from build123d import *

# Parameters (mm, degrees)
SKETCH_1_W          = 70
SKETCH_1_H          = 30
EXTRUDE_1_DEPTH     = 2
SKETCH_2_R          = 5
EXTRUDE_2_DEPTH     = 4
SKETCH_3_W          = 100
SKETCH_3_H          = 20
EXTRUDE_3_DEPTH     = 4
EXTRUDE_5_DEPTH     = 100
SKETCH_7_W          = 40
SKETCH_7_H          = 30
EXTRUDE_7_DEPTH     = 6
CUT_EXTRUDE_1_REACH = 97
SKETCH_8_R          = 1.5
CUT_EXTRUDE_2_REACH = 95.814
SKETCH_10_R         = 14


with BuildPart() as part:
    # 草图1 → 凸台-拉伸1 (new body)
    with BuildSketch(Plane(origin=(0, 0, 0), x_dir=(1, 0, 0), z_dir=(0, 1, 0))):
        with Locations((35, 15)):
            Rectangle(SKETCH_1_W, SKETCH_1_H)
    extrude(amount=EXTRUDE_1_DEPTH)

    # 草图2 → 凸台-拉伸2 (add)
    with BuildSketch(Plane(origin=(0, 0, 0), x_dir=(1, 0, 0), z_dir=(0, 1, 0))):
        with Locations(Location((5, 25, 0), (0, 0, 90))):
            Circle(SKETCH_2_R)
        with Locations(Location((5, 5, 0), (0, 0, 270))):
            Circle(SKETCH_2_R)
        with Locations(Location((65, 25, 0), (0, 0, 90))):
            Circle(SKETCH_2_R)
        with Locations(Location((65, 5, 0), (0, 0, 270))):
            Circle(SKETCH_2_R)
    extrude(amount=EXTRUDE_2_DEPTH)

    # 草图3 → 凸台-拉伸3 (add)
    with BuildSketch(Plane(origin=(0, 0, -30), x_dir=(-1, 0, 0), z_dir=(0, 0, -1))):
        with Locations((-35, -10)):
            Rectangle(SKETCH_3_W, SKETCH_3_H)
    extrude(amount=-EXTRUDE_3_DEPTH)

    # 草图5 → 凸台-拉伸5 (add)
    with BuildSketch(Plane.ZY.offset(15)):
        Polygon((-30, 0), (-35, -10), (-30, -20), align=None)
    extrude(amount=-EXTRUDE_5_DEPTH)

    # 草图7 → 凸台-拉伸7 (add)
    with BuildSketch(Plane.XY.offset(-11)):
        with Locations((35, -15)):
            Rectangle(SKETCH_7_W, SKETCH_7_H)
    extrude(amount=EXTRUDE_7_DEPTH)

    # 草图8 → 切除-拉伸1 (cut, up to next)
    with BuildSketch(Plane.XY.offset(-5), mode=Mode.PRIVATE) as cut_extrude_1_sk1:
        with Locations((23, -3)):
            Circle(SKETCH_8_R)
    cut_extrude_1_tool1 = extrude(cut_extrude_1_sk1.sketch, amount=-CUT_EXTRUDE_1_REACH, mode=Mode.PRIVATE) & part.part
    # 草图8 → 切除-拉伸1 (cut, up to next)
    with BuildSketch(Plane.XY.offset(-5), mode=Mode.PRIVATE) as cut_extrude_1_sk2:
        with Locations((47, -3)):
            Circle(SKETCH_8_R)
    cut_extrude_1_tool2 = extrude(cut_extrude_1_sk2.sketch, amount=-CUT_EXTRUDE_1_REACH, mode=Mode.PRIVATE) & part.part
    # 草图8 → 切除-拉伸1 (cut, up to next)
    with BuildSketch(Plane.XY.offset(-5), mode=Mode.PRIVATE) as cut_extrude_1_sk3:
        with Locations((23, -27)):
            Circle(SKETCH_8_R)
    cut_extrude_1_tool3 = extrude(cut_extrude_1_sk3.sketch, amount=-CUT_EXTRUDE_1_REACH, mode=Mode.PRIVATE) & part.part
    # 草图8 → 切除-拉伸1 (cut, up to next)
    with BuildSketch(Plane.XY.offset(-5), mode=Mode.PRIVATE) as cut_extrude_1_sk4:
        with Locations((47, -27)):
            Circle(SKETCH_8_R)
    cut_extrude_1_tool4 = extrude(cut_extrude_1_sk4.sketch, amount=-CUT_EXTRUDE_1_REACH, mode=Mode.PRIVATE) & part.part
    add(cut_extrude_1_tool1.solids().sort_by_distance((23, -3, -5))[0], mode=Mode.SUBTRACT)
    add(cut_extrude_1_tool2.solids().sort_by_distance((47, -3, -5))[0], mode=Mode.SUBTRACT)
    add(cut_extrude_1_tool3.solids().sort_by_distance((23, -27, -5))[0], mode=Mode.SUBTRACT)
    add(cut_extrude_1_tool4.solids().sort_by_distance((47, -27, -5))[0], mode=Mode.SUBTRACT)

    # 草图10 → 切除-拉伸2 (cut, up to next)
    with BuildSketch(Plane.XY.offset(-26), mode=Mode.PRIVATE) as cut_extrude_2_sk1:
        with Locations((35, -15)):
            Circle(SKETCH_10_R)
    cut_extrude_2_tool1 = extrude(cut_extrude_2_sk1.sketch, amount=-CUT_EXTRUDE_2_REACH, mode=Mode.PRIVATE) & part.part
    add(cut_extrude_2_tool1.solids().sort_by_distance((35, -15, -26))[0], mode=Mode.SUBTRACT)


solid = part.part
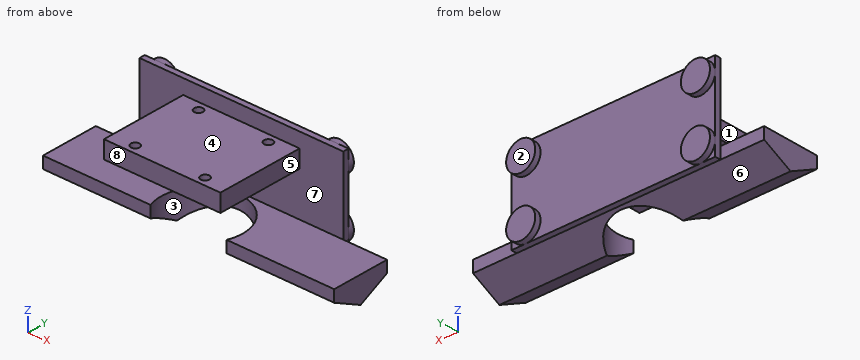
Verification items for the finished model (mm, model axes). Face numbers are marked on the shaded views. A direction names the side the tool comes from. Round coordinates to 2 decimals unless told otherwise and drop trailing zeros. Loops run counter-clockwise (first coordinate to the right, second up) from the corner with the lowest first, then second, coordinate; pieces in that order, holes last. Notation, with made-up numbers: (41.5, -26.5) - (65.5, -26.5) arc R21 cw to (65.5, 5.5) - close; hole circle Ø1 at (70, 1). An arc over 180 degrees is marked (long way). Use one line per item in the form item = value.
1. Section check C-C on x = 27. Record the cut outline in (y, z).
A:
outline = (-30, -11) - (0, -11) - (0, -26) - (-3.51, -26) - (-3.51, -31.76) - (0, -30) - (2, -30) - (2, 0) - (0, 0) - (0, -5) - (-30, -5) - close
2. Gauge pin test, flat ends, axial feed: pin 1 Ø6 at (x, z) = (23, -4) entering from +Y; pin 2 Ø12 at (x, z) = (18, -30) entering from -Y; pin 3 Ø2 at (x, z) = (-11, -28.5) entering from +Y. Record the tip position at first contact, or that the pin passes through.
A:
pin_1 = 2
pin_2 = -20
pin_3 = 0
3. Draft check along Z on the marked faces 6, 7 and 8. Enter one of: pulls with the +Z half, pulls with the -Z half, needs draft (parallel to the pull), parting line crosses it, or undercut.
A:
face_6 = pulls with the -Z half
face_7 = undercut
face_8 = needs draft
4. Section check B-B on y = -18. Record the cut outline in (x, z).
A:
outline = (-15, -31) - (21.33, -31) - (21.33, -26) - (-15, -26) - close; (15, -11) - (55, -11) - (55, -5) - (15, -5) - close; (48.67, -31) - (85, -31) - (85, -26) - (48.67, -26) - close
5. Access from +Z, -Z, +X, -X, +Y, -Y to the whole of each face (thin tool, end or side, straight path). Record for the marked faces 1, 2, 3, 4 and 5.
A:
face_1 = +Z, -X, -Y
face_2 = +Z, -Z, +X, -X, +Y
face_3 = -Z
face_4 = +Z, +X, -X, -Y
face_5 = +Z, +X, -Y
6. Section check A-A on z = -22. Record the cut outline in (x, y).
A:
outline = (0, 0) - (70, 0) - (70, 2) - (69, 2) - (69, 4) - (61, 4) - (61, 2) - (9, 2) - (9, 4) - (1, 4) - (1, 2) - (0, 2) - close
7. Section check D-D on y = -24. Record the cut outline in (x, z).
A:
outline = (15, -11) - (55, -11) - (55, -5) - (15, -5) - close
8. Scan lines: probe 1 along X at (y, z) = (-15, -29); probe 2 along Z at (x, y) = (51, -10); probe 3 along Y at (x, z) = (1, -12.5). Record each from-to range of solid material in increasing order.
A:
probe_1 = -15 to 21, 49 to 85
probe_2 = -35 to -26, -11 to -5
probe_3 = 0 to 2
